Can you work these out from the model? Positions are in its coordinate system, mm. Face numbers are marked on the shaded views. A direction names the side the tool comes from. Give positions to 0.01 mm unless a question says otherwise; leave off trailing zeros. Loops run counter-clockwise (first coordinate to the right, second up) from the corner with the lowest first, then second, coordinate; pieces in that order, holes last. Notation, with made-up numbers: (12, -21.75) -> (60, -21.75) arc R24 ccw to (60, -9.75) -> close; hole circle Ø4 at (14, 84.5). An arc over 180 degrees is marked (long way). Use CSV: the item, a comma, the result in double quotes.
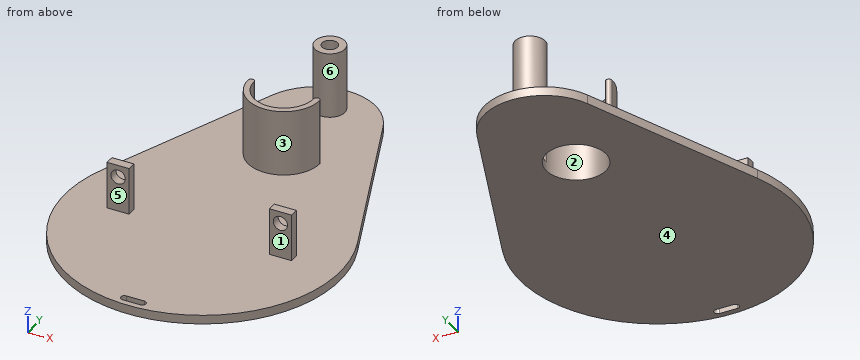
from build123d import *

# Parameters (mm, degrees)
PAD018_DEPTH    = 1.5
SKETCH025_R     = 2.5
SKETCH025_R_2   = 1.3
PAD019_DEPTH    = 11
SKETCH030_R     = 5
POCKET010_DEPTH = 5
PAD022_DEPTH    = 11
SKETCH032_W     = 3.7
SKETCH032_H     = 7.9
SKETCH032_R     = 1.2
PAD023_DEPTH    = 1.5


with BuildPart() as part:
    # Sketch024 (on XY_Plane011 of Origin022) → Pad018 (new body)
    with BuildSketch(Plane.XY):
        with BuildLine():
            ThreePointArc((9.284615, 3.714286), (0, 10), (-9.284615, 3.714286))
            Line((-9.284615, 3.714286), (-21.354615, -26.457143))
            ThreePointArc((-21.354615, -26.457143), (0, -58), (21.354615, -26.457143))
            Line((9.284615, 3.714286), (21.354615, -26.457143))
        make_face()
        with BuildLine():
            ThreePointArc((-1.5, -55.8), (-2.1, -56.4), (-1.5, -57))
            Line((-1.5, -57), (1.5, -57))
            ThreePointArc((1.5, -57), (2.1, -56.4), (1.5, -55.8))
            Line((-1.5, -55.8), (1.5, -55.8))
        make_face(mode=Mode.SUBTRACT)
    extrude(amount=PAD018_DEPTH)

    # Sketch025 (on Face10 of Pad018) → Pad019 (join)
    with BuildSketch(Plane.XY.offset(1.5)):
        with Locations((-0.057612, 4.499631)):
            Circle(SKETCH025_R)
        with Locations((-0.057612, 4.499631)):
            Circle(SKETCH025_R_2, mode=Mode.SUBTRACT)
    extrude(amount=PAD019_DEPTH)

    # Sketch030 (on Face5 of Pad021) → Pocket010 (cut)
    with BuildSketch(Plane.XY.offset(1.5)):
        with Locations((0, -9.825034)):
            Circle(SKETCH030_R)
    extrude(amount=-POCKET010_DEPTH, mode=Mode.SUBTRACT)

    # Sketch031 (on Face5 of Pocket010) → Pad022 (join)
    with BuildSketch(Plane.XY.offset(1.5)):
        with BuildLine():
            ThreePointArc((-6, -9.825034), (0, -15.825034), (6, -9.825034))
            ThreePointArc((6, -9.825034), (5.5, -9.325034), (5, -9.825034))
            ThreePointArc((-5, -9.825034), (0, -14.825034), (5, -9.825034))
            ThreePointArc((-5, -9.825034), (-5.5, -9.325034), (-6, -9.825034))
        make_face()
    pad022 = extrude(amount=PAD022_DEPTH)

    # Mirrored003: Pad022 across Sketch031 V_Axis
    add(pad022.mirror(Plane(origin=(0, 0, 1.5), x_dir=(0, 0, 1), z_dir=(1, 0, 0))))

    # Sketch032 (on Face2 of Binder008) → Pad023 (join)
    with BuildSketch(Plane(origin=(0, -35.550008, 0), x_dir=(-1, 0, 0), z_dir=(0, 1, 0))):
        with Locations((-13.35, 5.45)):
            Rectangle(SKETCH032_W, SKETCH032_H)
        with Locations((-13.35, 7.4)):
            Circle(SKETCH032_R, mode=Mode.SUBTRACT)
        with Locations((13.85, 5.45)):
            Rectangle(SKETCH032_W, SKETCH032_H)
        with Locations((13.85, 7.4)):
            Circle(SKETCH032_R, mode=Mode.SUBTRACT)
    extrude(amount=PAD023_DEPTH)


solid = part.part
(1) If we section it at C-C, the plane x = -13.85: Write out the boundary of the cut face in (y, z), then the cut area to 3 significant figures.
Answer sheet:
outline,"(-53.36, 0) -> (-7.7, 0) -> (-7.7, 1.5) -> (-34.05, 1.5) -> (-34.05, 6.2) -> (-35.55, 6.2) -> (-35.55, 1.5) -> (-53.36, 1.5) -> close; (-35.55, 8.6) -> (-34.05, 8.6) -> (-34.05, 9.4) -> (-35.55, 9.4) -> close"
area,"76.7 mm2"
(2) If we section it at B-B, the plane y = -5.5: Write out the boundary of the cut face in (x, z), then the cut area to 3 significant figures.
Answer sheet:
outline,"(-12.97, 0) -> (-2.51, 0) -> (-2.51, 1.5) -> (-12.97, 1.5) -> close; (2.51, 0) -> (12.97, 0) -> (12.97, 1.5) -> (2.51, 1.5) -> close"
area,"31.4 mm2"
(3) If I drill on L1, parallel to Y at x = 1, z = 4; L2, parallel to Z at x = 0, y = 0.5; L3, parallel to X at y = -35.5, z = 3.25, over which ranges is the centre line in solid material (lowest first)? Write a range as from..to.
Answer sheet:
L1,"y = -15.74..-14.72, 2.23..3.74, 5.26..6.76"
L2,"z = 0..1.5"
L3,"x = -15.7..-12, 11.5..15.2"
(4) Which directions (+Z, -Z, +X, -X, +Y, -Y) give clear straight access to the entire face, cutting with the end or side of a thin tool? Please do the marked faces 1, 2 and 3.
Answer sheet:
face 1,"+Z, +X, -X, -Y"
face 2,"+Z, -Z"
face 3,"+Z, -Y"
(5) Will these pins go through, and if not, where does the flat tip stop? pin 1 Ø5 at (x, z) = (-12, 8) entering from +Y; pin 2 Ø8 at (x, y) = (0, -9.83) entering from +Z; pin 3 Ø1.2 at (y, z) = (-34.5, 3.5) entering from +X; pin 4 Ø6 at (x, z) = (-4, 3) entering from -Y.
Answer sheet:
pin 1,"stops at y = -34.05"
pin 2,"passes through"
pin 3,"stops at x = 15.2"
pin 4,"stops at y = -57.96"
(6) If we section it at A-A, the plane z = 5: Write out the boundary of the cut face in (x, y), then the cut area to 3 significant figures.
Answer sheet:
outline,"(-15.7, -35.55) -> (-12, -35.55) -> (-12, -34.05) -> (-15.7, -34.05) -> close; (-6, -9.83) arc R6 ccw to (6, -9.83) arc R0.5 ccw to (5, -9.83) arc R5 cw to (-5, -9.83) arc R0.5 ccw to start; circle Ø5 at (-0.06, 4.5); (11.5, -35.55) -> (15.2, -35.55) -> (15.2, -34.05) -> (11.5, -34.05) -> close; hole circle Ø2.6 at (-0.06, 4.5)"
area,"43.5 mm2"
(7) We'd pull the mould along Y, two halves only. Please class the marked faces 4, 5 and 6: released by +Y, released by -Y, zero draft, split by the parting line, or undercut.
Answer sheet:
face 4,"zero draft"
face 5,"released by -Y"
face 6,"undercut"
(8) If we section it at D-D, the plane z = 10.75: Write out the boundary of the cut face in (x, y).
Answer sheet:
outline,"(-6, -9.83) arc R6 ccw to (6, -9.83) arc R0.5 ccw to (5, -9.83) arc R5 cw to (-5, -9.83) arc R0.5 ccw to start; circle Ø5 at (-0.06, 4.5); hole circle Ø2.6 at (-0.06, 4.5)"
